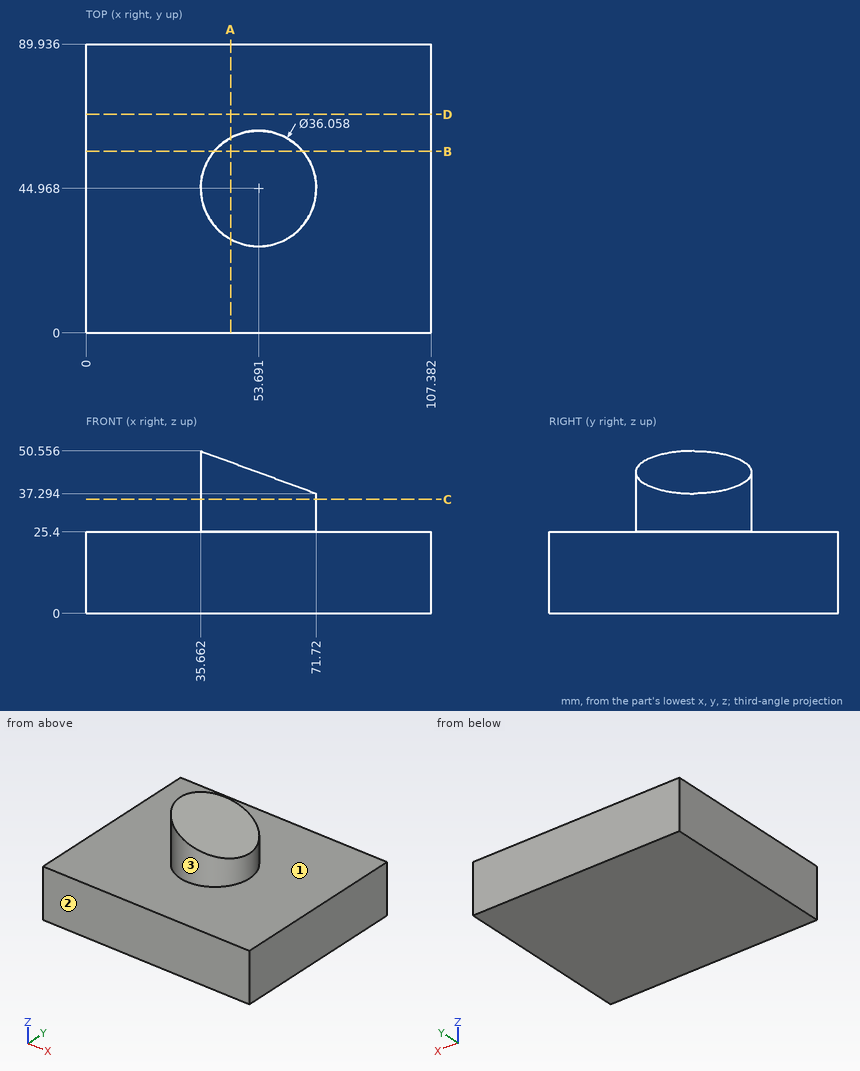
The figure shows three views and two pictorial views of one solid part (mm, origin at its lowest corner). Answer the questions. Round coordinates to 2 decimals unless told otherwise and drop trailing zeros. Order: outer loops, then holes, each group sorted by start corner. A loop starts at its lowest first (then second) coordinate and runs counter-clockwise, first axis right, second up. Notation, with made-up numbers: (63.25, -9.75) -> (71.25, -9.75) arc R21 ccw to (71.25, 1.25) -> close; hole circle Ø7 at (25, 14). An arc over 180 degrees is marked (long way). Put each result on its own line as item: value.
Q1. Section A-A, the plane x = 45 is taken. Write down the section's boundary in (y, z), and give its area (3 significant figures).
Results list:
outline: (0, 0) -> (89.94, 0) -> (89.94, 25.4) -> (60.76, 25.4) -> (60.76, 47.12) -> (29.17, 47.12) -> (29.17, 25.4) -> (0, 25.4) -> close
area: 2,970 mm^2
Q2. Section C-C, the plane z = 35.5 is taken. Write down the section's boundary in (x, y), and give its area (3 significant figures).
Results list:
outline: circle Ø36.06 at (53.69, 44.97)
area: 1,020 mm^2
Q3. Section B-B, the plane y = 56.5 is taken. Write down the section's boundary in (x, z).
Results list:
outline: (0, 0) -> (107.38, 0) -> (107.38, 25.4) -> (67.55, 25.4) -> (67.55, 38.83) -> (39.83, 49.02) -> (39.83, 25.4) -> (0, 25.4) -> close
Q4. Section D-D, the plane y = 68 is taken. Write down the section's boundary in (x, z).
Results list:
outline: (0, 0) -> (107.38, 0) -> (107.38, 25.4) -> (0, 25.4) -> close
Q5. Each of these flat-tipped pins is pushed along its axis until it touches: P1, Ø10, axis at y = 38, z = 26.5, coming from the +X side; P2, Ø1.5, axis at x = 57.5, y = 48.5, coming from the +Z side; P3, Ø1, axis at x = 62, z = 32.5, coming from the -Y side; P4, Ø4, axis at x = 92, y = 13.5, coming from the +Z side. Where does it stop, or does it pass through?
Results list:
P1: x = 107.38
P2: z = 42.8
P3: y = 28.72
P4: z = 25.4
Q6. Consider line 1 along Z through (x, y) = (77, 8); line 2 along Y through (x, z) = (39, 44); line 3 along Z through (x, y) = (46.5, 46). Determine where each line is inside the solid, lowest interval first.
Results list:
line 1: 0 to 25.4
line 2: 34.52 to 55.42
line 3: 0 to 46.57
Q7. Determine the mould class of the marked faces 1, 2 and 3 for opening direction Y: pulls with the +Y half, pulls with the -Y half, needs draft (parallel to the pull), parting line crosses it, or undercut.
Results list:
face 1: needs draft
face 2: pulls with the -Y half
face 3: parting line crosses it
